For this review, use the dimensioned drawing (mm, ordinates from the lowest corner) and the shaded views. A direction names the side the tool comes from. Round coordinates to 2 decimals unless told otherwise and drop trailing zeros. Write each loop counter-clockwise with the first axis right and the second up, starting at its lowest first coordinate (ties: lowest second). Pieces come first, ordered by that corner, then holes. Notation, with made-up numbers: M 31,69 L 55,69 A19 ccw 55,85 Z; hole C -19,-16 d8. An arc over 180 degrees is marked long. One line per question, with ' | ' between items. Start each with the question number.
Item 1: For L1, parallel to X at y = 65.5, z = 484.5; L2, parallel to Y at x = 49.5, z = 39; L3, parallel to Y at x = 535, z = 46.5 (1 decimal), list the stretches that pass through material, from the lowest coordinate up.
Item 2: Add section C-C, the plane x = 313. State the section outline as (y, z) points.
Item 3: Add section B-B, the plane z = 399. State the section outline as (x, y) points (3 decimals), and give its area (3 significant figures).
Item 4: Machinability: for the marked faces 4, 5, 6, 7 and 8, which of the approach directions +Z, -Z, +X, -X, +Y, -Y give a long, thin tool a straight path to every point of the face, cutting with its end or side? Answer none if there is none.
Item 5: Draft analysis for pull direction Y (two halves, no side actions). For the marked faces 1, 2 and 3, state which applies: released by +Y, released by -Y, zero draft, split by the parting line, or undercut.
Item 6: Insertion check: pin 1 Ø8 at (x, z) = (399, 233.5) entering from +Y; pin 2 Ø10 at (y, z) = (380, 212.5) entering from +X; pin 3 Ø6 at (x, y) = (149, 308.5) entering from +Z. Each pin has a flat end and moves straight along its axis. Give the tip position at first contact, or say it passes through.
Item 7: Add section A-A, the plane y = 367.5. State the section outline as (x, z) points.
Item 8: Add section D-D, the plane y = 182.5. State the section outline as (x, z) points, and give its area (3 significant figures).
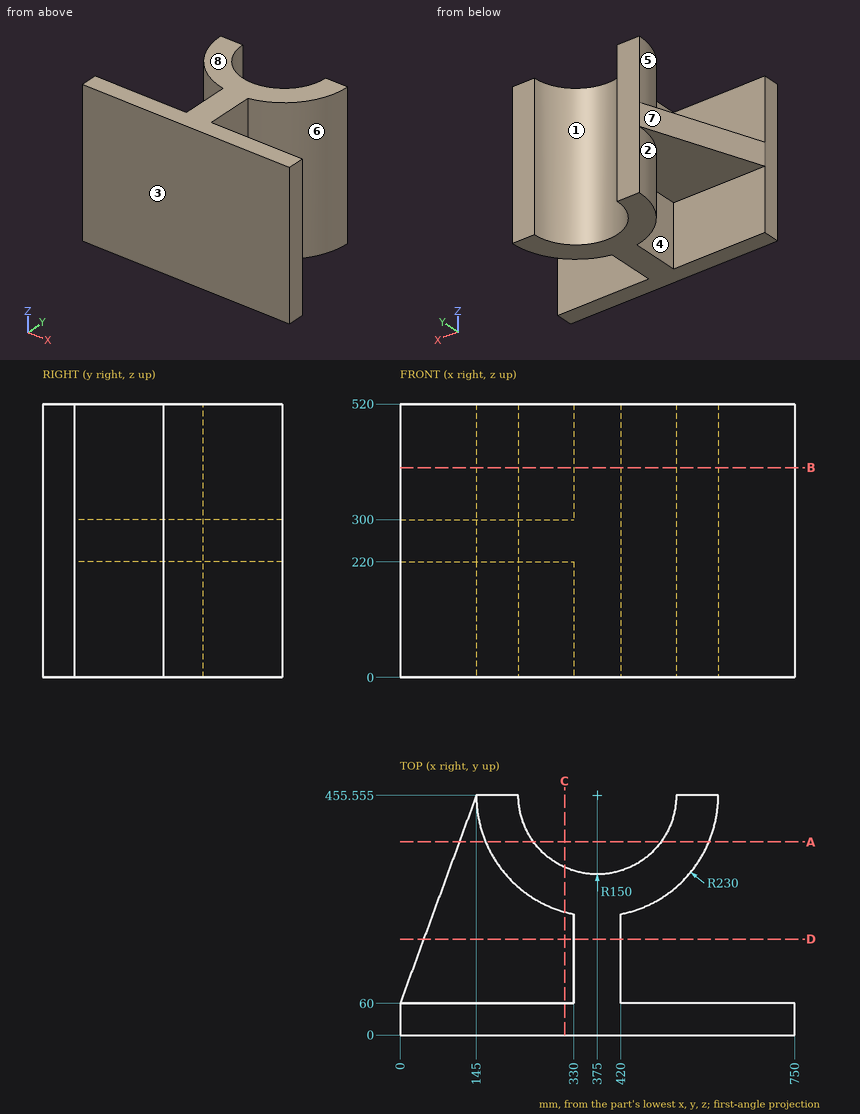
Computed values:
1) L1: x = 330 to 420 | L2: y = 0 to 60 | L3: y = 0 to 60, 290.3 to 455.6
2) outline: M 0,0 L 60,0 L 60,220 L 234.07,220 L 234.07,0 L 318.97,0 L 318.97,520 L 234.07,520 L 234.07,300 L 60,300 L 60,520 L 0,520 Z
3) outline: M 0,0 L 750,0 L 750,60 L 420,60 L 420,230 A230 ccw 605,455.555 L 525,455.555 A150 cw 225,455.555 L 145,455.555 A230 ccw 330,230 L 330,60 L 0,60 Z | area: 108,000 mm^2
4) face 4: -Z, -X | face 5: +Z, -X | face 6: +Z, -Z, +X | face 7: +Z, -Z, -X, +Y | face 8: +Z, +X, -X, +Y, -Y
5) face 1: released by +Y | face 2: undercut | face 3: released by -Y
6) pin 1: stops at y = 308.19 | pin 2: stops at x = 593.91 | pin 3: stops at z = 300
7) outline: M 112.72,220 L 162.52,220 L 162.52,0 L 253.57,0 L 253.57,520 L 162.52,520 L 162.52,300 L 112.72,300 Z; M 496.43,0 L 587.48,0 L 587.48,520 L 496.43,520 Z
8) outline: M 44.91,220 L 330,220 L 330,0 L 420,0 L 420,520 L 330,520 L 330,300 L 44.91,300 Z | area: 69,600 mm^2
